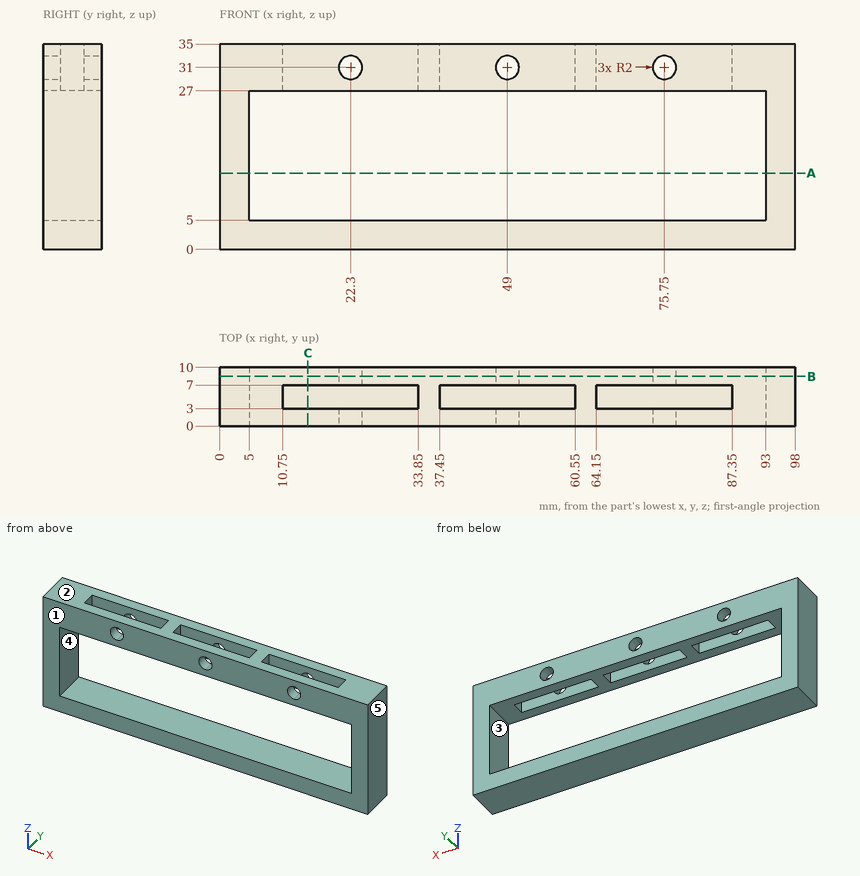
Can you work these out from the drawing? Everything is in mm from the part's minimum corner. A direction names the side the tool comes from. Round coordinates to 2 decimals unless told otherwise and drop trailing zeros. Write each loop counter-clockwise with the first axis right and the second up, starting at its lowest first coordinate (ties: lowest second). Pieces come first, ordered by that corner, then holes. Notation, with made-up numbers: (40.25, 20.25) - (44.25, 20.25) arc R22 cw to (44.25, 27.25) - close; hole circle Ø2 at (26.5, 9.5). An arc over 180 degrees is marked (long way). Use a Markdown table: item, result.
Q1. I want a section at B-B (y = 8.5). List the corners of the cut face in (x, z) for me.
Output values:
| item | result |
|---|---|
| outline | (0, 0) - (98, 0) - (98, 35) - (0, 35) - close; hole (5, 5) - (93, 5) - (93, 27) - (5, 27) - close; hole circle Ø4 at (22.3, 31); hole circle Ø4 at (49, 31); hole circle Ø4 at (75.75, 31) |
Q2. For the marked faces 4 and 5, which set-ups out of +Z, -Z, +X, -X, +Y, -Y let a thin tool reach every point of the face, with its end or its side?
Output values:
| item | result |
|---|---|
| face 4 | +Y, -Y |
| face 5 | +Z, -Z, +X, +Y, -Y |
Q3. Please list where these lines run through material, in increasing order: L1, parallel to X at y = 6.5, z = 29; L2, parallel to Y at x = 69, z = 32; L3, parallel to X at y = 1.25, z = 20.5.
Output values:
| item | result |
|---|---|
| L1 | 0 to 10.75, 33.85 to 37.45, 60.55 to 64.15, 87.35 to 98 |
| L2 | 0 to 3, 7 to 10 |
| L3 | 0 to 5, 93 to 98 |
Q4. For pin 1 (2.5 mm diameter, centred on x = 16.5, z = 32.5, fed in from -Y); pin 2 (2.5 mm diameter, centred on x = 22.5, z = 31, fed in from +Y), each with a flat end and sliding along its axis, tell me the tip position at first contact or that it passes through.
Output values:
| item | result |
|---|---|
| pin 1 | y = 0 |
| pin 2 | through |
Q5. Thinking about a two-plate mould opening in Z: for the marked faces 1, 2 and 3, which applies, released by +Z, released by -Z, zero draft, split by the parting line, or undercut?
Output values:
| item | result |
|---|---|
| face 1 | zero draft |
| face 2 | released by +Z |
| face 3 | undercut |
Q6. I want a section at C-C (x = 15). List the corners of the cut face in (y, z) for me.
Output values:
| item | result |
|---|---|
| outline | (0, 0) - (10, 0) - (10, 5) - (0, 5) - close; (0, 27) - (3, 27) - (3, 35) - (0, 35) - close; (7, 27) - (10, 27) - (10, 35) - (7, 35) - close |
Q7. I want a section at A-A (z = 13). List the corners of the cut face in (x, y) for me.
Output values:
| item | result |
|---|---|
| outline | (0, 0) - (5, 0) - (5, 10) - (0, 10) - close; (93, 0) - (98, 0) - (98, 10) - (93, 10) - close |
